Job drawing, mm, ordinate dimensions from the low corner. One solid piece. A direction names the side the tool comes from. Give positions to 0.01 mm unless a question says otherwise; leave off trailing zeros. Order: outer loops, then holes, each group sorted by start corner. A loop starts at its lowest first (then second) coordinate and runs counter-clockwise, first axis right, second up. Notation, with made-up numbers: (69.5, 22.25) - (73.5, 22.25) arc R22 ccw to (73.5, 36.25) - close; hole circle Ø4 at (65.5, 40.5). An arc over 180 degrees is marked (long way). Write each question's results on one line, items separated by ' | '. Start each with the question number.
1) Tool access for the marked faces 1, 2 and 3: list every direction of +Z, -Z, +X, -X, +Y, -Y with a clear straight run to the whole face (end or side of a thin tool).
2) Cut at C-C on z = 6.5. List the corners of the cut face in (x, y), plus the area to 3 significant figures.
3) Cut at D-D on x = 50.5. List the corners of the cut face in (y, z).
4) Drill centre lines: line 1 along Y through (x, z) = (6.35, 4.5); line 2 along Y through (x, z) = (6, 4) (1 decimal); line 3 along X through (y, z) = (35, 21). Where is each one in solid material? Low to high. Write a range as from..to.
5) Drop flat-ended pins along their axis: pin 1 Ø5 at (y, z) = (15.5, 38.5) entering from +X; pin 2 Ø4 at (y, z) = (5.5, 29.5) entering from -X; pin 3 Ø3 at (x, y) = (4.5, 11.5) entering from +Z. Give the stop position or say it passes through.
6) Two-plate mould, pull along X, no slides. Class the marked faces 4, 5, 6 and 7: +X half, -X half, draft (parallel to the pull), parting line (faces both ways), or undercut.
7) Cut at B-B on y = 22.5. List the corners of the cut face in (x, z).
8) Cut at A-A on x = 6.35. List the corners of the cut face in (y, z).
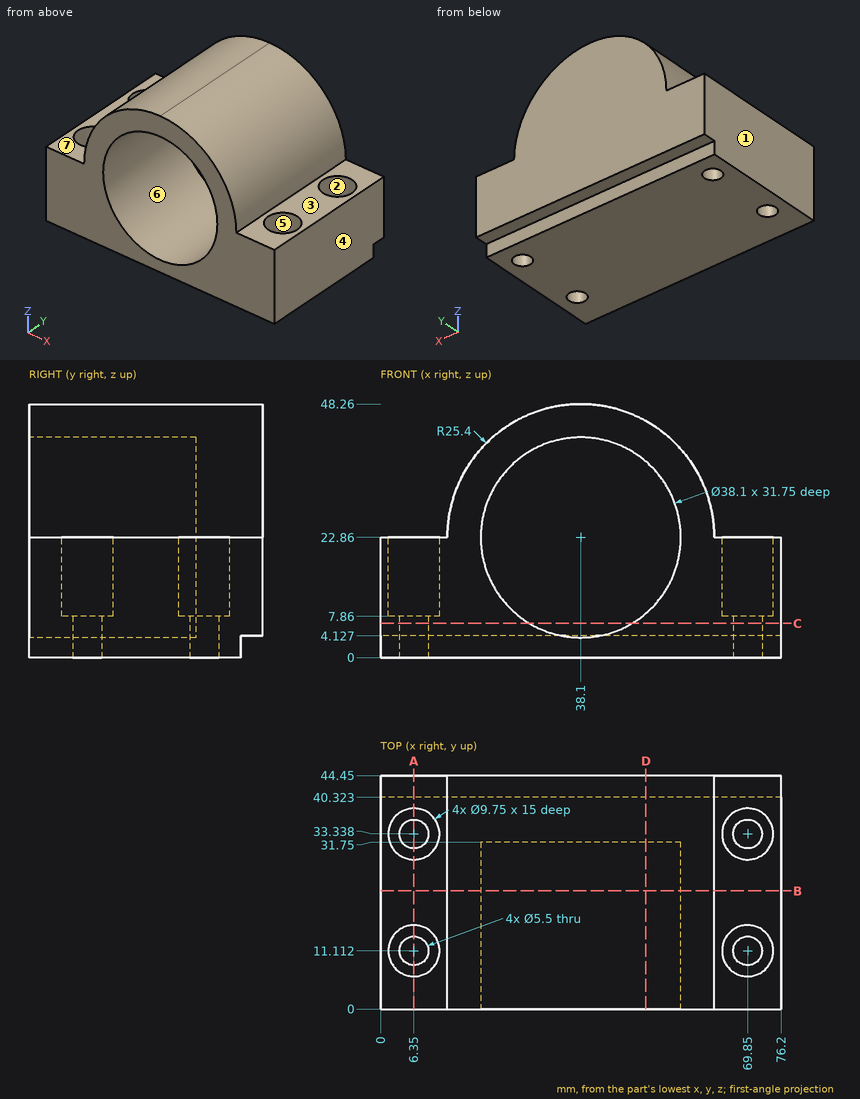
Results:
1) face 1: +Z, -Z, -X, +Y, -Y | face 2: +Z | face 3: +Z, +X, +Y, -Y
2) outline: (0, 0) - (28.34, 0) - (28.34, 31.75) - (47.86, 31.75) - (47.86, 0) - (76.2, 0) - (76.2, 44.45) - (0, 44.45) - close; hole circle Ø5.5 at (6.35, 11.11); hole circle Ø5.5 at (6.35, 33.34); hole circle Ø5.5 at (69.85, 11.11); hole circle Ø5.5 at (69.85, 33.34) | area: 2,670 mm^2
3) outline: (0, 0) - (40.32, 0) - (40.32, 4.13) - (44.45, 4.13) - (44.45, 45.03) - (0, 45.03) - (0, 37.32) - (31.75, 37.32) - (31.75, 8.4) - (0, 8.4) - close
4) line 1: 0..8.36, 13.86..30.59, 36.09..44.45 | line 2: 0..8.4, 13.8..30.6, 36.1..40.3 | line 3: 0..1.77, 10.93..65.27, 74.43..76.2
5) pin 1: x = 59.84 | pin 2: x = 13.13 | pin 3: z = 7.86
6) face 4: +X half | face 5: undercut | face 6: undercut | face 7: draft
7) outline: (0, 0) - (76.2, 0) - (76.2, 22.86) - (63.5, 22.86) arc R25.4 ccw to (12.7, 22.86) - (0, 22.86) - close; hole circle Ø38.1 at (38.1, 22.86)
8) outline: (0, 0) - (8.36, 0) - (8.36, 7.86) - (6.24, 7.86) - (6.24, 22.86) - (0, 22.86) - close; (13.86, 0) - (30.59, 0) - (30.59, 7.86) - (28.46, 7.86) - (28.46, 22.86) - (15.99, 22.86) - (15.99, 7.86) - (13.86, 7.86) - close; (36.09, 0) - (40.32, 0) - (40.32, 4.13) - (44.45, 4.13) - (44.45, 22.86) - (38.21, 22.86) - (38.21, 7.86) - (36.09, 7.86) - close
